The drawing under review shows one solid part. Ordinate dimensions are in mm from its lowest x, y, z. Give positions to 0.01 mm unless a question says otherwise; leave off trailing zeros. Write each loop counter-clockwise with the first axis right and the second up, starting at its lowest first coordinate (ties: lowest second). Pieces come first, ordered by that corner, then holes. Notation, with made-up numbers: (28.25, -19) - (51.25, -19) arc R27 cw to (51.25, 18) - close; hole circle Ø2 at (13, -22). An arc over 180 degrees is marked (long way). Write item = value, one per line.
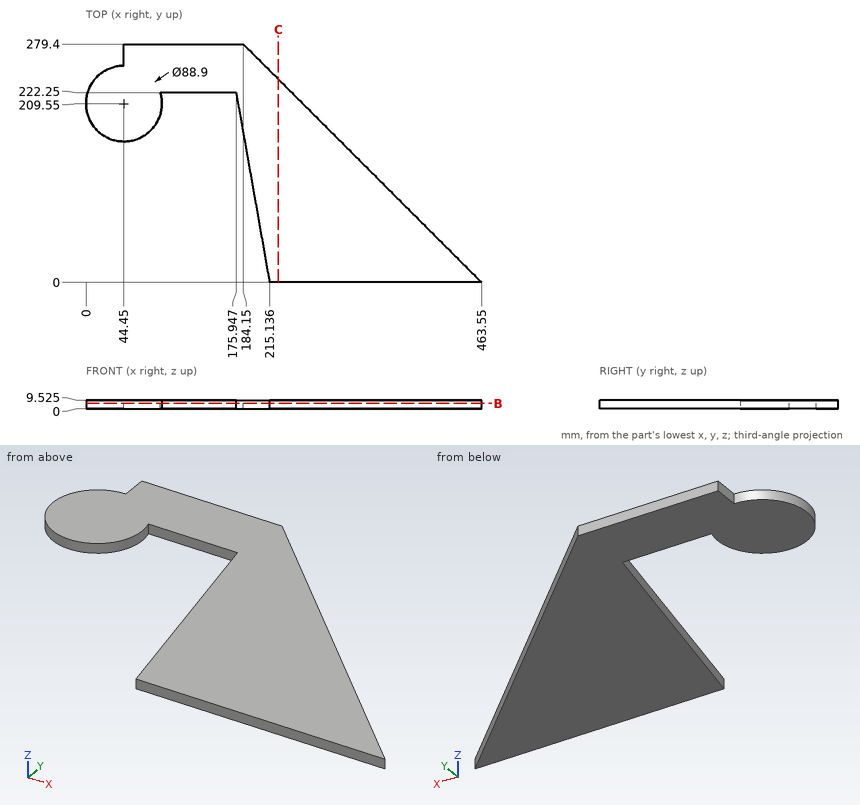
1. Insertion check: P1, Ø3, axis at x = 113, z = 7, coming from the -Y side; P2, Ø1.5, axis at x = 333, z = 7.5, coming from the +Y side; P3, Ø5, axis at x = 50.5, z = 3.5, coming from the -Y side. Each pin has a flat end and moves straight along its axis. Give the tip position at first contact, or say it passes through.
Findings below:
P1 = 222.25
P2 = 131.3
P3 = 165.24
2. For line 1 (Y direction, x = 149, z = 4.5); line 2 (X direction, y = 179, z = 7.25); line 3 (X direction, y = 150, z = 0.75), list the stretches that pass through material, from the lowest coordinate up. Write a range as from..to.
Findings below:
line_1 = 222.25..279.4
line_2 = 12.16..76.74, 183.57..284.55
line_3 = 188.69..313.55
3. Take a section at C-C on x = 225.5. Give the boundary of the cut face in (y, z) (3 decimals).
Findings below:
outline = (0, 0) - (238.05, 0) - (238.05, 9.525) - (0, 9.525) - close
4. Take a section at B-B on z = 6. Give the boundary of the cut face in (x, y), and give its area (3 significant figures).
Findings below:
outline = (44.45, 254) arc R44.45 ccw (long way) to (87.05, 222.25) - (175.95, 222.25) - (215.14, 0) - (463.55, 0) - (184.15, 279.4) - (44.45, 279.4) - close
area = 49,700 mm²
